```python
from build123d import *

# Parameters (mm, degrees)
F1_DEPTH = 1701.8


with BuildPart() as f1:
    # F0 (on Top) → F1 (new body)
    with BuildSketch(Plane.XY):
        with BuildLine():
            ThreePointArc((0, 12.596164), (-1.859872, 17.086292), (-6.35, 18.946164))
            Line((-6.35, 18.946164), (-31.75, 18.946164))
            ThreePointArc((-31.75, 18.946164), (-36.240128, 17.086292), (-38.1, 12.596164))
            Line((-38.1, 12.596164), (-38.1, -12.803836))
            ThreePointArc((-38.1, -12.803836), (-36.240128, -17.293964), (-31.75, -19.153836))
            Line((-31.75, -19.153836), (-6.35, -19.153836))
            ThreePointArc((-6.35, -19.153836), (-1.859872, -17.293964), (0, -12.803836))
            Line((0, -12.803836), (0, -12.7))
            Line((0, -12.7), (0, 12.596164))
        make_face()
        with BuildLine():
            Line((0, 12.7), (0, 12.596164))
            Line((0, 12.596164), (0, -12.7))
            ThreePointArc((0, -12.7), (1.859872, -17.190128), (6.35, -19.05))
            Line((6.35, -19.05), (31.75, -19.05))
            ThreePointArc((31.75, -19.05), (36.240128, -17.190128), (38.1, -12.7))
            Line((38.1, -12.7), (38.1, 12.7))
            ThreePointArc((38.1, 12.7), (36.240128, 17.190128), (31.75, 19.05))
            Line((31.75, 19.05), (6.35, 19.05))
            ThreePointArc((6.35, 19.05), (1.859872, 17.190128), (0, 12.7))
        make_face()
    extrude(amount=F1_DEPTH)


solid = f1.part
```
Check sheet for the modelled part. Datum: model origin and axes. Units: mm. Round coordinates to 2 decimals unless told otherwise and drop trailing zeros. Order: outer loops, then holes, each group sorted by start corner. A loop starts at its lowest first (then second) coordinate and runs counter-clockwise, first axis right, second up. Notation, with made-up numbers: (70, 81.5) -> (82, 81.5) arc R31 cw to (82, 113.5) -> close; hole circle Ø2 at (32, 67). An arc over 180 degrees is marked (long way). Use CSV: the item, a comma, the result in double quotes.
(1) Material ranges on line 1 along Y through (x, z) = (-17, 298); line 2 along Y through (x, z) = (9.5, 1598); line 3 along X through (y, z) = (15.5, 1448.5), recorded low to high. Write a range as from..to.
Worked out:
line 1,"-19.15..18.95"
line 2,"-19.05..19.05"
line 3,"-37.4..-0.7, 0.65..37.45"
(2) Cross-section at A-A (z = 1490). Record the boundary of the cut face in (x, y).
Worked out:
outline,"(-38.1, -12.8) arc R6.35 ccw to (-31.75, -19.15) -> (-6.35, -19.15) arc R6.35 ccw to (0, -12.8) -> (0, -12.7) arc R6.35 ccw to (6.35, -19.05) -> (31.75, -19.05) arc R6.35 ccw to (38.1, -12.7) -> (38.1, 12.7) arc R6.35 ccw to (31.75, 19.05) -> (6.35, 19.05) arc R6.35 ccw to (0, 12.7) -> (0, 12.6) arc R6.35 ccw to (-6.35, 18.95) -> (-31.75, 18.95) arc R6.35 ccw to (-38.1, 12.6) -> close"
(3) Depth check by flat-ended pin: pin 1 (7.5 mm diameter, centred on x = 21, z = 1011.5, fed in from -Y); pin 2 (7.5 mm diameter, centred on x = -18.5, z = 909, fed in from +Y). Enter the tip coordinate at first touch or a pass-through.
Worked out:
pin 1,"y = -19.05"
pin 2,"y = 18.95"
